from build123d import *

# Parameters (mm, degrees)
F1_DEPTH = 25.4
F3_DEPTH = 31.75
F5_DEPTH = 25.908


with BuildPart() as f1:
    # F0 (on Front) → F1 (new body)
    with BuildSketch(Plane.XZ):
        Polygon((0, 31.75), (0, 0), (38.1, 0), (38.1, 6.35), (12.7, 6.35), (12.7, 31.75), align=None)
    extrude(amount=F1_DEPTH)

    # F2 (on Top) → F3 (join)
    with BuildSketch(Plane.XY):
        Polygon((0, 6.35), (0, 0), (0, -25.4), (12.7, -25.4), (12.7, 0), (38.1, 0), (38.1, 6.35), align=None)
    extrude(amount=F3_DEPTH)

    # F4 (on face) → F5 (join)
    with BuildSketch(Plane.YZ.offset(38.1)):
        Polygon((0, 31.75), (-25.4, 6.35), (0, 6.35), align=None)
    extrude(amount=-F5_DEPTH)


solid = f1.part
Read the model definition and answer for the solid it produces. Units are mm, in the model's axes. A direction names the side the tool comes from. Give positions to 0.01 mm unless a question says otherwise; leave off trailing zeros. Write each loop counter-clockwise with the first axis right and the second up, starting at its lowest first coordinate (ties: lowest second). Pieces come first, ordered by that corner, then holes. Notation, with made-up numbers: (-28.5, -4) -> (-12.5, -4) arc R17 cw to (-12.5, 0) -> close; hole circle Ø2 at (51, 32). An arc over 180 degrees is marked (long way). Answer as a JSON object with one key per item and string values. Group by question number.
1) Each of these flat-tipped pins is pushed along its axis until it touches: P1, Ø1, axis at x = 15.5, y = -17, coming from the +Z side; P2, Ø6, axis at x = 31.5, z = 14, coming from the -Y side. Where does it stop, or does it pass through?
2) Find section B-B (y = -18). Write down the section's boundary in (x, z), and give its area (3 significant figures).
3) Find section A-A (z = 29.5). Write down the section's boundary in (x, y), and give its area (3 significant figures).
4) A tool of negligible diameter and unlimited length cuts with its end or side. For faces 1 (the flat face through (19, -9, 0)), 2 (the flat face through (12.7, -18, 25)), from which of +Z, -Z, +X, -X, +Y, -Y can it reach the whole face along a straight path? Write none if from no direction.
5) Find section C-C (x = 28). Write down the section's boundary in (y, z), and give its area (3 significant figures).
6) Consider L1, parallel to Z at x = 30, y = -12; L2, parallel to Z at x = 30.5, y = -6; L3, parallel to Y at x = 18, z = 17. Determine where each line is inside the solid, lowest interval first. Write a range as from..to.
Values follow:
{
 "1": {"P1": "stops at z = 15.25", "P2": "stops at y = -20.75"},
 "2": {"outline": "(0, 0) -> (38.1, 0) -> (38.1, 13.75) -> (12.7, 13.75) -> (12.7, 31.75) -> (0, 31.75) -> close", "area": "752 mm2"},
 "3": {"outline": "(0, -25.4) -> (12.7, -25.4) -> (12.7, -2.25) -> (38.1, -2.25) -> (38.1, 6.35) -> (0, 6.35) -> close", "area": "622 mm2"},
 "4": {"face 1": "-Z, +X, -X, +Y, -Y", "face 2": "+Z, +X, -Y"},
 "5": {"outline": "(-25.4, 0) -> (6.35, 0) -> (6.35, 31.75) -> (0, 31.75) -> (-25.4, 6.35) -> close", "area": "685 mm2"},
 "6": {"L1": "z = 0..19.75", "L2": "z = 0..25.75", "L3": "y = -14.75..6.35"}
}
